Build history of the part. All positions in model axes, mm. Face numbers are marked on the shaded views. A direction names the side the tool comes from. Give positions to 0.01 mm unless a question says otherwise; leave off trailing zeros. Order: outer loops, then holes, each group sorted by start corner. A loop starts at its lowest first (then second) coordinate and runs counter-clockwise, first axis right, second up. Notation, with made-up numbers: (21.25, 33.25) - (25.25, 33.25) arc R8 cw to (25.25, 43.25) - close; hole circle Ø1 at (-38, 65). An arc over 180 degrees is marked (long way). Use a Markdown table: item, result.
from build123d import *

# Parameters (mm, degrees)
SKETCH1_R               = 1.525
SKETCH1_R_2             = 2.5
SKETCH1_R_3             = 1.5
MAIN_BODY_DEPTH         = 10
SKETCH1_4_R             = 2.5
LEAD_SCREW_CUTOUT_DEPTH = 40.593410121
LIMIT_SWITCH_TAB_DEPTH  = 17
CUT_EXTRUDE1_DEPTH      = 42.912266999
FILLET1_R               = 0.6
CHAMFER1_SIZE           = 0.6
CUT_EXTRUDE2_DEPTH      = 3.8
CUT_EXTRUDE3_DEPTH      = 49.211668712
CUT_EXTRUDE4_DEPTH      = 3.3


with BuildPart() as part:
    # Sketch1 → Main body (new body)
    # profile 1 of 3: a face of its own
    with BuildSketch(Plane(origin=(0, 0, 0), x_dir=(1, 0, 0), z_dir=(0, 1, 0))):
        with BuildLine():
            Line((18.75, 6.525), (-18.75, 6.525))
            Line((-18.75, 6.525), (-35.75, 6.525))
            ThreePointArc((-35.75, 6.525), (-37.164213562, 5.939213562), (-37.75, 4.525))
            Line((-37.75, 4.525), (-37.75, -4.525))
            ThreePointArc((-37.75, -4.525), (-37.164213562, -5.939213562), (-35.75, -6.525))
            Line((-35.75, -6.525), (-18.75, -6.525))
            Line((-18.75, -6.525), (18.75, -6.525))
            ThreePointArc((18.75, -6.525), (25.275, 0), (18.75, 6.525))
        make_face()
        with Locations(Location((-18.75, 0, 0), (0, 0, 270))):
            Circle(SKETCH1_R, mode=Mode.SUBTRACT)
        Circle(SKETCH1_R_2, mode=Mode.SUBTRACT)
        with Locations(Location((18.75, 0, 0), (0, 0, 270))):
            Circle(SKETCH1_R, mode=Mode.SUBTRACT)
    # profile 2 of 3: a face of its own
    with BuildSketch(Plane(origin=(0, 0, 0), x_dir=(1, 0, 0), z_dir=(0, 1, 0))):
        Circle(SKETCH1_R_2)
        Circle(SKETCH1_R_3, mode=Mode.SUBTRACT)
    # profile 3 of 3: a face of its own
    with BuildSketch(Plane(origin=(0, 0, 0), x_dir=(1, 0, 0), z_dir=(0, 1, 0))):
        Circle(SKETCH1_R_3)
    extrude(amount=MAIN_BODY_DEPTH)

    # Sketch1<4> → Lead screw cutout (cut, through all)
    with BuildSketch(Plane(origin=(0, 0, 0), x_dir=(1, 0, 0), z_dir=(0, 1, 0))):
        with Locations(Location((0, 0, 0), (0, 0, 270))):
            Circle(SKETCH1_4_R)
    extrude(amount=LEAD_SCREW_CUTOUT_DEPTH, mode=Mode.SUBTRACT)

    # Limit switch tab sketch → Limit switch tab (add)
    with BuildSketch(Plane(origin=(0, 10, 0), x_dir=(1, 0, 0), z_dir=(0, 1, 0))):
        with BuildLine():
            Line((-37.75, 4.525), (-37.75, -4.525))
            ThreePointArc((-37.75, -4.525), (-37.164213562, -5.939213562), (-35.75, -6.525))
            Line((-35.75, -6.525), (-31.75, -6.525))
            ThreePointArc((-31.75, -6.525), (-30.335786438, -5.939213562), (-29.75, -4.525))
            Line((-29.75, -4.525), (-29.75, 4.525))
            ThreePointArc((-29.75, 4.525), (-30.335786438, 5.939213562), (-31.75, 6.525))
            Line((-31.75, 6.525), (-35.75, 6.525))
            ThreePointArc((-35.75, 6.525), (-37.164213562, 5.939213562), (-37.75, 4.525))
        make_face()
    extrude(amount=LIMIT_SWITCH_TAB_DEPTH)

    # Sketch2 → Cut-Extrude1 (cut, through all)
    with BuildSketch(Plane(origin=(0, 10, 0), x_dir=(1, 0, 0), z_dir=(0, 1, 0))):
        with BuildLine():
            Line((-27.25, 0.5), (27.993605311, 0.5))
            Line((27.993605311, 0.5), (27.993605311, -0.5))
            Line((27.993605311, -0.5), (-27.25, -0.5))
            ThreePointArc((-27.25, -0.5), (-27.75, 0), (-27.25, 0.5))
        make_face()
    extrude(amount=-CUT_EXTRUDE1_DEPTH, mode=Mode.SUBTRACT)

    # Fillet1
    fillet1_edges = [part.edges().sort_by_distance(p)[0] for p in [
        (2.449489743, 5, 0.5),
        (-2.449489743, 5, 0.5),
        (-2.449489743, 5, -0.5),
        (2.449489743, 5, -0.5),
        (-17.309297047, 5, -0.5),
        (-20.190702953, 5, -0.5),
        (20.190702953, 5, -0.5),
        (17.309297047, 5, -0.5),
        (25.255814707, 5, -0.5),
        (-20.190702953, 5, 0.5),
        (-17.309297047, 5, 0.5),
        (17.309297047, 5, 0.5),
        (20.190702953, 5, 0.5),
        (25.255814707, 5, 0.5),
    ]]
    fillet(fillet1_edges, radius=FILLET1_R)

    # Chamfer1
    chamfer1_edges = [part.edges().sort_by_distance(p)[0] for p in [
        (22.913609585, 0, -5.023940706),
        (-8.5, 0, 6.525),
        (-37.164213562, 0, 5.939213562),
        (-37.75, 0, 0),
        (9.915068783, 10, -0.5),
        (9.915068783, 0, -0.5),
        (22.570066358, 0, -0.5),
        (-37.164213562, 0, -5.939213562),
        (18.75, 0, -1.525),
        (0, 0, -2.5),
        (-9.915068783, 0, -0.5),
        (-18.75, 0, -1.525),
        (-23.909068892, 0, -0.5),
        (-18.75, 0, 1.525),
        (-9.915068783, 0, 0.5),
        (0, 0, 2.5),
        (-8.5, 0, -6.525),
        (9.915068783, 0, 0.5),
        (18.75, 0, 1.525),
        (22.570066358, 0, 0.5),
        (22.913609585, 0, 5.023940706),
        (-20.273479457, 0, -0.577337135),
        (-17.226520543, 0, -0.577337135),
        (-20.273479457, 0, 0.577337135),
        (-17.226520543, 0, 0.577337135),
        (-2.557498249, 0, 0.606167065),
        (-2.557498249, 0, -0.606167065),
        (2.557498249, 0, 0.606167065),
        (17.226520543, 0, -0.577337135),
        (17.226520543, 0, 0.577337135),
        (20.273479457, 0, 0.577337135),
        (20.273479457, 0, -0.577337135),
        (25.033966492, 0, -0.717139348),
        (25.033966492, 0, 0.717139348),
        (2.557498249, 0, -0.606167065),
        (0, 10, -2.5),
        (22.570066358, 10, -0.5),
        (22.913609585, 10, 5.023940706),
        (22.570066358, 10, 0.5),
        (18.75, 10, 1.525),
        (9.915068783, 10, 0.5),
        (0, 10, 2.5),
        (-9.915068783, 10, 0.5),
        (-18.75, 10, 1.525),
        (-23.909068892, 10, -0.5),
        (-18.75, 10, -1.525),
        (-9.915068783, 10, -0.5),
        (18.75, 10, -1.525),
        (-20.273479457, 10, -0.577337135),
        (-17.226520543, 10, -0.577337135),
        (-20.273479457, 10, 0.577337135),
        (-17.226520543, 10, 0.577337135),
        (-2.557498249, 10, 0.606167065),
        (-2.557498249, 10, -0.606167065),
        (2.557498249, 10, 0.606167065),
        (17.226520543, 10, -0.577337135),
        (17.226520543, 10, 0.577337135),
        (20.273479457, 10, 0.577337135),
        (20.273479457, 10, -0.577337135),
        (25.033966492, 10, -0.717139348),
        (25.033966492, 10, 0.717139348),
        (2.557498249, 10, -0.606167065),
        (-6.5, 10, -6.525),
        (-6.5, 10, 6.525),
        (-37.164213562, 27, 5.939213562),
        (-33.75, 27, 6.525),
        (-30.335786438, 27, 5.939213562),
        (-29.75, 27, 0),
        (-30.335786438, 27, -5.939213562),
        (-33.75, 27, -6.525),
        (-37.164213562, 27, -5.939213562),
        (-37.75, 27, 0),
        (22.913609585, 10, -5.023940706),
        (-23.909068892, 0, 0.5),
        (-27.75, 0, 0),
        (-27.75, 10, 0),
        (-23.909068892, 10, 0.5),
    ]]
    chamfer(chamfer1_edges, length=CHAMFER1_SIZE - 0.0001)  # a hair under: the kernel refuses the full size

    # Sketch3 → Cut-Extrude2 (cut)
    # profile 1 of 2: a face of its own
    with BuildSketch(Plane.XY.offset(6.525)):
        Polygon((12.2, 3.36898549), (12.2, 6.63101451), (9.375, 8.262029021), (6.55, 6.63101451), (6.55, 3.36898549), (9.375, 1.737970979), align=None)
        with BuildLine():
            ThreePointArc((8.346539825, 6.225671109), (9.375, 3.4), (10.403460175, 6.225671109))
            Line((10.403460175, 6.225671109), (9.375, 7.088651663))
            Line((9.375, 7.088651663), (8.346539825, 6.225671109))
        make_face(mode=Mode.SUBTRACT)
    # profile 2 of 2: a face of its own
    with BuildSketch(Plane.XY.offset(6.525)):
        with BuildLine():
            Line((9.375, 7.088651663), (8.346539825, 6.225671109))
            ThreePointArc((8.346539825, 6.225671109), (9.375, 3.4), (10.403460175, 6.225671109))
            Line((10.403460175, 6.225671109), (9.375, 7.088651663))
        make_face()
    extrude(amount=-CUT_EXTRUDE2_DEPTH, mode=Mode.SUBTRACT)

    # Sketch3<3> → Cut-Extrude3 (cut, through all)
    with BuildSketch(Plane.XY.offset(6.525)):
        with BuildLine():
            Line((9.375, 7.088651663), (8.346539825, 6.225671109))
            ThreePointArc((8.346539825, 6.225671109), (9.375, 3.4), (10.403460175, 6.225671109))
            Line((10.403460175, 6.225671109), (9.375, 7.088651663))
        make_face()
    extrude(amount=-CUT_EXTRUDE3_DEPTH, mode=Mode.SUBTRACT)

    # Sketch4 → Cut-Extrude4 (cut)
    with BuildSketch(Plane(origin=(0, 0, -6.525), x_dir=(-1, 0, 0), z_dir=(0, 0, -1))):
        with BuildLine():
            Line((-9.375, 8.687775592), (-11.190874997, 7.164075552))
            ThreePointArc((-11.190874997, 7.164075552), (-9.375, 2.175), (-7.559125003, 7.164075552))
            Line((-7.559125003, 7.164075552), (-9.375, 8.687775592))
        make_face()
    extrude(amount=-CUT_EXTRUDE4_DEPTH, mode=Mode.SUBTRACT)


solid = part.part
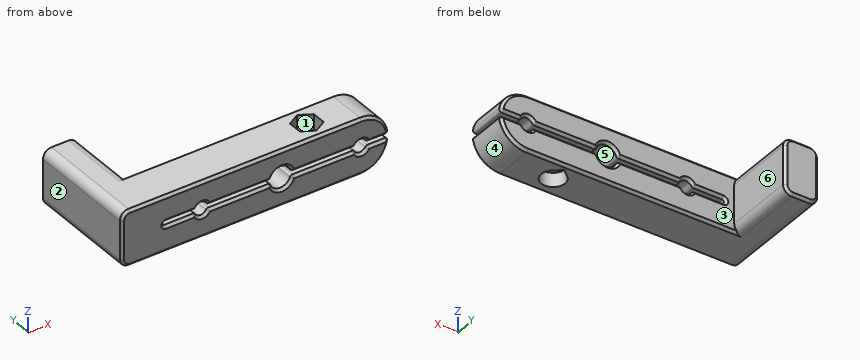
1) Tool access for the marked faces 4, 5 and 6: list every direction of +Z, -Z, +X, -X, +Y, -Y with a clear straight run to the whole face (end or side of a thin tool).
Computed:
| item | result |
|---|---|
| face 4 | -Z, +X, +Y, -Y |
| face 5 | +Y, -Y |
| face 6 | +Z, -Z, +X, +Y |
2) Slice it at B-B (y = 14.5). Write the cut outline in (x, z) (3 decimals).
Computed:
| item | result |
|---|---|
| outline | (-37.75, -4.525) arc R2 ccw to (-35.75, -6.525) - (-31.75, -6.525) arc R2 ccw to (-29.75, -4.525) - (-29.75, 4.525) arc R2 ccw to (-31.75, 6.525) - (-35.75, 6.525) arc R2 ccw to (-37.75, 4.525) - close |
3) Pin check, flat tips, straight feed: P1, Ø3, axis at x = 15, z = 3, coming from the +Y side; P2, Ø4, axis at x = -23.5, y = 12.5, coming from the -Z side; P3, Ø5, axis at x = 9.375, y = 5, coming from the -Z side (3 decimals); P4, Ø3.5, axis at x = 9.375, y = 5, coming from the +Z side (3 decimals). Stop position of each tip, or through.
Computed:
| item | result |
|---|---|
| P1 | stops at y = 10 |
| P2 | passes through |
| P3 | stops at z = -3.225 |
| P4 | stops at z = 2.725 |
4) Wall check: line 1 (Z direction, x = -7, y = 7.5) (3 decimals); line 2 (X direction, y = 5, z = 2.1) (3 decimals); line 3 (X direction, y = 5, z = 1.95) (3 decimals). Give the ranges that are in metal, low to high. Write a range as from..to.
Computed:
| item | result |
|---|---|
| line 1 | z = -6.525..-0.5, 0.5..6.525 |
| line 2 | x = -37.75..-1.356, 1.356..7.775, 10.975..24.928 |
| line 3 | x = -37.75..-1.564, 1.564..7.775, 10.975..24.977 |
5) Slice it at C-C (y = 5). State how many separate pieces and enclosed holes the cut face has, and give its area (3 significant figures).
Computed:
| item | result |
|---|---|
| separate pieces | 3 |
| enclosed holes | 0 |
| area | 670 mm² |
6) Slice it at A-A (x = -10). Write the cut outline in (y, z) (3 decimals), and give its area (3 significant figures).
Computed:
| item | result |
|---|---|
| outline | (0, -5.925) - (0.6, -6.525) - (9.4, -6.525) - (10, -5.925) - (10, -1.1) - (9.4, -0.5) - (0.6, -0.5) - (0, -1.1) - close; (0, 1.1) - (0.6, 0.5) - (9.4, 0.5) - (10, 1.1) - (10, 5.925) - (9.4, 6.525) - (0.6, 6.525) - (0, 5.925) - close |
| area | 119 mm² |
7) Two-plate mould, pull along X, no slides. Class the marked faces 1, 2 and 3: +X half, -X half, draft (parallel to the pull), parting line (faces both ways), or undercut.
Computed:
| item | result |
|---|---|
| face 1 | undercut |
| face 2 | -X half |
| face 3 | draft |
